CAD build for the part. Positions are in the model's coordinates, mm. Give positions to 0.01 mm unless a question says otherwise; leave off trailing zeros. Loops run counter-clockwise (first coordinate to the right, second up) from the corner with the lowest first, then second, coordinate; pieces in that order, holes last.
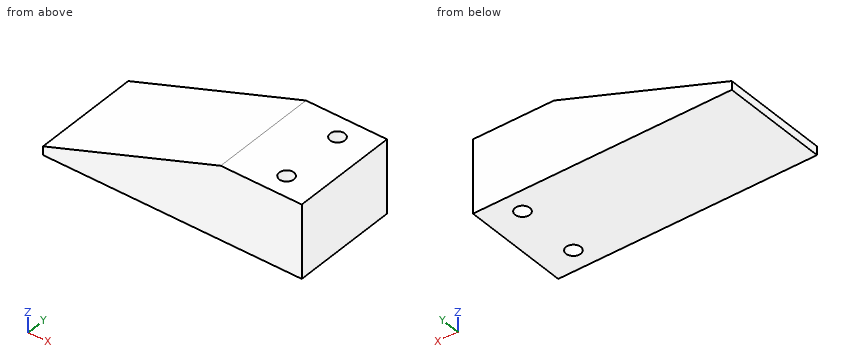
```python
from build123d import *

# Parameters (mm, degrees)
BOSS_EXTRUDE1_DEPTH      = 8.5
BOSS_EXTRUDE1_DEPTH_BACK = 8.5
SKETCH2_R                = 1.7
CHAMFER1_SIZE            = 15
CHAMFER1_SIZE2           = 41.212161292


with BuildPart() as part:
    # Sketch2 → Boss-Extrude1 (new, two sides: drawn at the far end of the back side and taken through both)
    with BuildSketch(Plane.XY.offset(-BOSS_EXTRUDE1_DEPTH_BACK)):
        Polygon((-7.5, 12.5), (7.5, 12.5), (7.5, -12.5), (-7.5, -12.5), (-52.5, -12.5), (-52.5, 12.5), align=None)
        with Locations((0, 7.466666667)):
            Circle(SKETCH2_R, mode=Mode.SUBTRACT)
        with Locations((0, -7.466666667)):
            Circle(SKETCH2_R, mode=Mode.SUBTRACT)
    extrude(amount=BOSS_EXTRUDE1_DEPTH + BOSS_EXTRUDE1_DEPTH_BACK)

    # Chamfer1
    chamfer1_edges = [part.edges().sort_by_distance(p)[0] for p in [
        (-52.5, 0, 8.5),
    ]]
    chamfer1_side = [part.faces().sort_by_distance(p)[0] for p in [
        (-52.5, 0, 0),
    ]]
    chamfer(chamfer1_edges, length=CHAMFER1_SIZE, length2=CHAMFER1_SIZE2, reference=chamfer1_side[0])


solid = part.part
```
1. Saw through at A-A, the plane x = 0. List the corners of the cut face in (y, z).
Responses:
outline: (-12.5, -8.5) - (-9.17, -8.5) - (-9.17, 8.5) - (-12.5, 8.5) - close; (-5.77, -8.5) - (5.77, -8.5) - (5.77, 8.5) - (-5.77, 8.5) - close; (9.17, -8.5) - (12.5, -8.5) - (12.5, 8.5) - (9.17, 8.5) - close
2. Saw through at D-D, the plane z = 4.25. List the corners of the cut face in (x, y).
Responses:
outline: (-22.96, -12.5) - (7.5, -12.5) - (7.5, 12.5) - (-22.96, 12.5) - close; hole circle Ø3.4 at (0, -7.47); hole circle Ø3.4 at (0, 7.47)
3. Saw through at B-B, the plane y = -1.75. List the corners of the cut face in (x, z).
Responses:
outline: (-52.5, -8.5) - (7.5, -8.5) - (7.5, 8.5) - (-11.29, 8.5) - (-52.5, -6.5) - close
4. Probe line 1 along Y through (x, z) = (0, -1); line 2 along Z through (x, y) = (-14, -7); line 3 along Y through (x, z) = (1, 4.75). List the from-to ranges inside material, lowest first.
Responses:
line 1: y = -12.5 to -9.17, -5.77 to 5.77, 9.17 to 12.5
line 2: z = -8.5 to 7.51
line 3: y = -12.5 to -8.84, -6.09 to 6.09, 8.84 to 12.5
5. Drop flat-ended pins along their axis: pin 1 (4 mm diameter, centred on x = -13.5, y = 9, fed in from +Z); pin 2 (3 mm diameter, centred on x = 0, y = 7.47, fed in from -Z); pin 3 (6 mm diameter, centred on x = -40, y = 0.5, fed in from +Z); pin 4 (4 mm diameter, centred on x = -20, y = 6.5, fed in from +Z). Give the stop position or say it passes through.
Responses:
pin 1: stops at z = 8.42
pin 2: passes through
pin 3: stops at z = -0.86
pin 4: stops at z = 6.06
6. Saw through at C-C, the plane z = 1. List the corners of the cut face in (x, y).
Responses:
outline: (-31.89, -12.5) - (7.5, -12.5) - (7.5, 12.5) - (-31.89, 12.5) - close; hole circle Ø3.4 at (0, -7.47); hole circle Ø3.4 at (0, 7.47)
